from build123d import *

# Parameters (mm, degrees)
EXTRUDE_THIN1_DEPTH       = 450
FILLET1_R                 = 1.2
CUT_EXTRUDE1_DEPTH        = 26
LPATTERN1_COUNT           = 17
LPATTERN1_PITCH           = 28
CIRPATTERN1_COUNT         = 2
CIRPATTERN1_ANGLE         = 270
CIRPATTERN1_COPY_1_DEPTH  = 26
CIRPATTERN1_COPY_2_DEPTH  = 26
CIRPATTERN1_COPY_3_DEPTH  = 26
CIRPATTERN1_COPY_4_DEPTH  = 26
CIRPATTERN1_COPY_5_DEPTH  = 26
CIRPATTERN1_COPY_6_DEPTH  = 26
CIRPATTERN1_COPY_7_DEPTH  = 26
CIRPATTERN1_COPY_8_DEPTH  = 26
CIRPATTERN1_COPY_9_DEPTH  = 26
CIRPATTERN1_COPY_10_DEPTH = 26
CIRPATTERN1_COPY_11_DEPTH = 26
CIRPATTERN1_COPY_12_DEPTH = 26
CIRPATTERN1_COPY_13_DEPTH = 26
CIRPATTERN1_COPY_14_DEPTH = 26
CIRPATTERN1_COPY_15_DEPTH = 26
CIRPATTERN1_COPY_16_DEPTH = 26
CUT_EXTRUDE2_DEPTH        = 4
SKETCH5_W                 = 23.8
SKETCH5_H                 = 25
CUT_EXTRUDE3_DEPTH        = 10


with BuildPart() as part:
    # Sketch1 → Extrude-Thin1 (new body)
    with BuildSketch(Plane(origin=(0, 0, 0), x_dir=(1, 0, 0), z_dir=(0, 1, 0))):
        Polygon((25, 0), (0, 0), (0, 25), (1.2, 25), (1.2, 1.2), (25, 1.2), align=None)
    extrude(amount=EXTRUDE_THIN1_DEPTH)

    # Fillet1
    fillet1_edges = [part.edges().sort_by_distance(p)[0] for p in [
        (0, 225, 0),
        (1.2, 225, -1.2),
    ]]
    fillet(fillet1_edges, radius=FILLET1_R)

    # Sketch2 → Cut-Extrude1 (cut, through all)
    with BuildSketch(Plane.XY):
        with BuildLine():
            Line((9, 9.5), (9, 16.5))
            ThreePointArc((9, 16.5), (12.5, 20), (16, 16.5))
            Line((16, 16.5), (16, 9.5))
            ThreePointArc((16, 9.5), (12.5, 6), (9, 9.5))
        make_face()
    cut_extrude1 = extrude(amount=-CUT_EXTRUDE1_DEPTH, mode=Mode.SUBTRACT)

    # LPattern1: Cut-Extrude1 ×17
    with Locations(*[(0, i * LPATTERN1_PITCH, 0) for i in range(1, LPATTERN1_COUNT)]):
        add(cut_extrude1, mode=Mode.SUBTRACT)

    # CirPattern1: Cut-Extrude1 ×2 about axis
    cirpattern1_axis = Axis((1.2, 450, 0), (0, -1, 0))
    for i in range(1, CIRPATTERN1_COUNT):
        add(cut_extrude1.rotate(cirpattern1_axis, i * CIRPATTERN1_ANGLE / (CIRPATTERN1_COUNT - 1)), mode=Mode.SUBTRACT)

    # CirPattern1 copy 1 sketch → CirPattern1 copy 1 (cut, through all)
    with BuildSketch(Plane(origin=(1.2, 28, 1.2), x_dir=(0, 0, -1), z_dir=(1, 0, 0))):
        with BuildLine():
            Line((9, 9.5), (9, 16.5))
            ThreePointArc((9, 16.5), (12.5, 20), (16, 16.5))
            Line((16, 16.5), (16, 9.5))
            ThreePointArc((16, 9.5), (12.5, 6), (9, 9.5))
        make_face()
    extrude(amount=-CIRPATTERN1_COPY_1_DEPTH, mode=Mode.SUBTRACT)

    # CirPattern1 copy 2 sketch → CirPattern1 copy 2 (cut, through all)
    with BuildSketch(Plane(origin=(1.2, 56, 1.2), x_dir=(0, 0, -1), z_dir=(1, 0, 0))):
        with BuildLine():
            Line((9, 9.5), (9, 16.5))
            ThreePointArc((9, 16.5), (12.5, 20), (16, 16.5))
            Line((16, 16.5), (16, 9.5))
            ThreePointArc((16, 9.5), (12.5, 6), (9, 9.5))
        make_face()
    extrude(amount=-CIRPATTERN1_COPY_2_DEPTH, mode=Mode.SUBTRACT)

    # CirPattern1 copy 3 sketch → CirPattern1 copy 3 (cut, through all)
    with BuildSketch(Plane(origin=(1.2, 84, 1.2), x_dir=(0, 0, -1), z_dir=(1, 0, 0))):
        with BuildLine():
            Line((9, 9.5), (9, 16.5))
            ThreePointArc((9, 16.5), (12.5, 20), (16, 16.5))
            Line((16, 16.5), (16, 9.5))
            ThreePointArc((16, 9.5), (12.5, 6), (9, 9.5))
        make_face()
    extrude(amount=-CIRPATTERN1_COPY_3_DEPTH, mode=Mode.SUBTRACT)

    # CirPattern1 copy 4 sketch → CirPattern1 copy 4 (cut, through all)
    with BuildSketch(Plane(origin=(1.2, 112, 1.2), x_dir=(0, 0, -1), z_dir=(1, 0, 0))):
        with BuildLine():
            Line((9, 9.5), (9, 16.5))
            ThreePointArc((9, 16.5), (12.5, 20), (16, 16.5))
            Line((16, 16.5), (16, 9.5))
            ThreePointArc((16, 9.5), (12.5, 6), (9, 9.5))
        make_face()
    extrude(amount=-CIRPATTERN1_COPY_4_DEPTH, mode=Mode.SUBTRACT)

    # CirPattern1 copy 5 sketch → CirPattern1 copy 5 (cut, through all)
    with BuildSketch(Plane(origin=(1.2, 140, 1.2), x_dir=(0, 0, -1), z_dir=(1, 0, 0))):
        with BuildLine():
            Line((9, 9.5), (9, 16.5))
            ThreePointArc((9, 16.5), (12.5, 20), (16, 16.5))
            Line((16, 16.5), (16, 9.5))
            ThreePointArc((16, 9.5), (12.5, 6), (9, 9.5))
        make_face()
    extrude(amount=-CIRPATTERN1_COPY_5_DEPTH, mode=Mode.SUBTRACT)

    # CirPattern1 copy 6 sketch → CirPattern1 copy 6 (cut, through all)
    with BuildSketch(Plane(origin=(1.2, 168, 1.2), x_dir=(0, 0, -1), z_dir=(1, 0, 0))):
        with BuildLine():
            Line((9, 9.5), (9, 16.5))
            ThreePointArc((9, 16.5), (12.5, 20), (16, 16.5))
            Line((16, 16.5), (16, 9.5))
            ThreePointArc((16, 9.5), (12.5, 6), (9, 9.5))
        make_face()
    extrude(amount=-CIRPATTERN1_COPY_6_DEPTH, mode=Mode.SUBTRACT)

    # CirPattern1 copy 7 sketch → CirPattern1 copy 7 (cut, through all)
    with BuildSketch(Plane(origin=(1.2, 196, 1.2), x_dir=(0, 0, -1), z_dir=(1, 0, 0))):
        with BuildLine():
            Line((9, 9.5), (9, 16.5))
            ThreePointArc((9, 16.5), (12.5, 20), (16, 16.5))
            Line((16, 16.5), (16, 9.5))
            ThreePointArc((16, 9.5), (12.5, 6), (9, 9.5))
        make_face()
    extrude(amount=-CIRPATTERN1_COPY_7_DEPTH, mode=Mode.SUBTRACT)

    # CirPattern1 copy 8 sketch → CirPattern1 copy 8 (cut, through all)
    with BuildSketch(Plane(origin=(1.2, 224, 1.2), x_dir=(0, 0, -1), z_dir=(1, 0, 0))):
        with BuildLine():
            Line((9, 9.5), (9, 16.5))
            ThreePointArc((9, 16.5), (12.5, 20), (16, 16.5))
            Line((16, 16.5), (16, 9.5))
            ThreePointArc((16, 9.5), (12.5, 6), (9, 9.5))
        make_face()
    extrude(amount=-CIRPATTERN1_COPY_8_DEPTH, mode=Mode.SUBTRACT)

    # CirPattern1 copy 9 sketch → CirPattern1 copy 9 (cut, through all)
    with BuildSketch(Plane(origin=(1.2, 252, 1.2), x_dir=(0, 0, -1), z_dir=(1, 0, 0))):
        with BuildLine():
            Line((9, 9.5), (9, 16.5))
            ThreePointArc((9, 16.5), (12.5, 20), (16, 16.5))
            Line((16, 16.5), (16, 9.5))
            ThreePointArc((16, 9.5), (12.5, 6), (9, 9.5))
        make_face()
    extrude(amount=-CIRPATTERN1_COPY_9_DEPTH, mode=Mode.SUBTRACT)

    # CirPattern1 copy 10 sketch → CirPattern1 copy 10 (cut, through all)
    with BuildSketch(Plane(origin=(1.2, 280, 1.2), x_dir=(0, 0, -1), z_dir=(1, 0, 0))):
        with BuildLine():
            Line((9, 9.5), (9, 16.5))
            ThreePointArc((9, 16.5), (12.5, 20), (16, 16.5))
            Line((16, 16.5), (16, 9.5))
            ThreePointArc((16, 9.5), (12.5, 6), (9, 9.5))
        make_face()
    extrude(amount=-CIRPATTERN1_COPY_10_DEPTH, mode=Mode.SUBTRACT)

    # CirPattern1 copy 11 sketch → CirPattern1 copy 11 (cut, through all)
    with BuildSketch(Plane(origin=(1.2, 308, 1.2), x_dir=(0, 0, -1), z_dir=(1, 0, 0))):
        with BuildLine():
            Line((9, 9.5), (9, 16.5))
            ThreePointArc((9, 16.5), (12.5, 20), (16, 16.5))
            Line((16, 16.5), (16, 9.5))
            ThreePointArc((16, 9.5), (12.5, 6), (9, 9.5))
        make_face()
    extrude(amount=-CIRPATTERN1_COPY_11_DEPTH, mode=Mode.SUBTRACT)

    # CirPattern1 copy 12 sketch → CirPattern1 copy 12 (cut, through all)
    with BuildSketch(Plane(origin=(1.2, 336, 1.2), x_dir=(0, 0, -1), z_dir=(1, 0, 0))):
        with BuildLine():
            Line((9, 9.5), (9, 16.5))
            ThreePointArc((9, 16.5), (12.5, 20), (16, 16.5))
            Line((16, 16.5), (16, 9.5))
            ThreePointArc((16, 9.5), (12.5, 6), (9, 9.5))
        make_face()
    extrude(amount=-CIRPATTERN1_COPY_12_DEPTH, mode=Mode.SUBTRACT)

    # CirPattern1 copy 13 sketch → CirPattern1 copy 13 (cut, through all)
    with BuildSketch(Plane(origin=(1.2, 364, 1.2), x_dir=(0, 0, -1), z_dir=(1, 0, 0))):
        with BuildLine():
            Line((9, 9.5), (9, 16.5))
            ThreePointArc((9, 16.5), (12.5, 20), (16, 16.5))
            Line((16, 16.5), (16, 9.5))
            ThreePointArc((16, 9.5), (12.5, 6), (9, 9.5))
        make_face()
    extrude(amount=-CIRPATTERN1_COPY_13_DEPTH, mode=Mode.SUBTRACT)

    # CirPattern1 copy 14 sketch → CirPattern1 copy 14 (cut, through all)
    with BuildSketch(Plane(origin=(1.2, 392, 1.2), x_dir=(0, 0, -1), z_dir=(1, 0, 0))):
        with BuildLine():
            Line((9, 9.5), (9, 16.5))
            ThreePointArc((9, 16.5), (12.5, 20), (16, 16.5))
            Line((16, 16.5), (16, 9.5))
            ThreePointArc((16, 9.5), (12.5, 6), (9, 9.5))
        make_face()
    extrude(amount=-CIRPATTERN1_COPY_14_DEPTH, mode=Mode.SUBTRACT)

    # CirPattern1 copy 15 sketch → CirPattern1 copy 15 (cut, through all)
    with BuildSketch(Plane(origin=(1.2, 420, 1.2), x_dir=(0, 0, -1), z_dir=(1, 0, 0))):
        with BuildLine():
            Line((9, 9.5), (9, 16.5))
            ThreePointArc((9, 16.5), (12.5, 20), (16, 16.5))
            Line((16, 16.5), (16, 9.5))
            ThreePointArc((16, 9.5), (12.5, 6), (9, 9.5))
        make_face()
    extrude(amount=-CIRPATTERN1_COPY_15_DEPTH, mode=Mode.SUBTRACT)

    # CirPattern1 copy 16 sketch → CirPattern1 copy 16 (cut, through all)
    with BuildSketch(Plane(origin=(1.2, 448, 1.2), x_dir=(0, 0, -1), z_dir=(1, 0, 0))):
        with BuildLine():
            Line((9, 9.5), (9, 16.5))
            ThreePointArc((9, 16.5), (12.5, 20), (16, 16.5))
            Line((16, 16.5), (16, 9.5))
            ThreePointArc((16, 9.5), (12.5, 6), (9, 9.5))
        make_face()
    extrude(amount=-CIRPATTERN1_COPY_16_DEPTH, mode=Mode.SUBTRACT)

    # Sketch3 → Cut-Extrude2 (cut)
    with BuildSketch(Plane(origin=(0, 450, 0), x_dir=(1, 0, 0), z_dir=(0, 1, 0))):
        with BuildLine():
            Line((0, 25), (0, 1.2))
            ThreePointArc((0, 1.2), (0.351471863, 0.351471863), (1.2, 0))
            Line((1.2, 0), (25, 0))
            Line((25, 0), (25, 1.2))
            Line((25, 1.2), (2.4, 1.2))
            ThreePointArc((2.4, 1.2), (1.551471863, 1.551471863), (1.2, 2.4))
            Line((1.2, 2.4), (1.2, 25))
            Line((1.2, 25), (0, 25))
        make_face()
    extrude(amount=-CUT_EXTRUDE2_DEPTH, mode=Mode.SUBTRACT)

    # Sketch5 → Cut-Extrude3 (cut)
    with BuildSketch(Plane.XY):
        with Locations((13.1, 433.5)):
            Rectangle(SKETCH5_W, SKETCH5_H)
        with Locations((13.1, 12.5)):
            Rectangle(SKETCH5_W, SKETCH5_H)
    extrude(amount=-CUT_EXTRUDE3_DEPTH, mode=Mode.SUBTRACT)


solid = part.part
Design review of the part built by this model. Coordinates are the model's own, in mm. A direction names the side the tool comes from. Coordinates: 2 decimals unless noted, no trailing zeros. Order: outer loops, then holes, each group sorted by start corner. A loop starts at its lowest first (then second) coordinate and runs counter-clockwise, first axis right, second up. Notation, with made-up numbers: (7.5, -15) -> (25.5, -15) arc R21 cw to (25.5, 4) -> close; hole circle Ø11 at (12.25, 31.5). An arc over 180 degrees is marked (long way). Use one line per item in the form item = value. Start each with the question number.
(1) For faces 1 (the flat face through (0, 220, -13)), 2 (the flat face through (14, 220, -1.2)), list the 3-axis set-ups (+Z, -Z, +X, -X, +Y, -Y) from which the entire face can be reached by the end or side of a thin tool; tool diameter is ignored.
(2) For probe 1 along Z at (x, y) = (21.5, 139); probe 2 along X at (y, z) = (114, -11.75); probe 3 along X at (y, z) = (137.5, -1.75), list the stretches that pass through material, from the lowest coordinate up.
(3) Add section A-A on y = 167. State the section outline as (x, z) points, plus the area to 3 significant figures.
(4) Insertion check: pin 1 (5 mm diameter, centred on y = 308, z = -8, fed in from +X); pin 2 (1.5 mm diameter, centred on x = 8.5, y = 173, fed in from -Z); pin 3 (3 mm diameter, centred on x = 3.5, z = -14.5, fed in from +Y); pin 4 (0.6 mm diameter, centred on x = 0.5, y = 97.5, fed in from +Z). Each pin has a flat end and moves straight along its axis. Give the tip position at first contact, or say it passes through.
(5) Add section B-B on z = -20.25. State the section outline as (x, y) points, plus the area to 3 significant figures.
Answer block:
q1.face_1 = +Z, -Z, -X, +Y, -Y
q1.face_2 = -Z, +X, +Y, -Y
q2.probe_1 = -1.2 to 0
q2.probe_2 = 0 to 1.2
q2.probe_3 = 0 to 1.39
q3.outline = (0, -25) -> (1.2, -25) -> (1.2, -2.4) arc R1.2 cw to (2.4, -1.2) -> (25, -1.2) -> (25, 0) -> (1.2, 0) arc R1.2 ccw to (0, -1.2) -> close
q3.area = 58.6 mm²
q4.pin_1 = 1.2
q4.pin_2 = -1.2
q4.pin_3 = through
q4.pin_4 = -0.07
q5.outline = (0, 0) -> (1.2, 0) -> (1.2, 446) -> (0, 446) -> close
q5.area = 535 mm²
